Could you check a few things on this model? Use its own coordinates, in mm. A direction names the side the tool comes from. Give positions to 0.01 mm unless a question says otherwise; leave off trailing zeros. Write each loop counter-clockwise with the first axis right and the second up, starting at its lowest first coordinate (ties: lowest second). Pieces come first, ordered by that corner, then holes. Notation, with made-up numbers: (-38, 28) - (-17, 28) arc R36 cw to (-17, 62) - close; hole circle Ø2 at (89, 89). An arc over 180 degrees is marked (long way). Write item = value, one per line.
from build123d import *

# Parameters (mm, degrees)
F0_R            = 2.15265
F1_DEPTH        = 12.7
F2_R            = 2.15265
F3_REACH        = 42.6021136501
F6_R            = 3.96875
F7_DEPTH        = 9.525
F9_DEPTH        = 12.7
F9_COPIES_COUNT = 3
F9_COPIES_ANGLE = 180
F10_R           = 3.96875
F11_DEPTH       = 9.525


# Not quite as in the source:
# - a pattern or mirror of a feature is missing from the dataset's text; its kind, count and spacing are read off the source's solid


with BuildPart() as f1:
    # F0 (on Top) → F1 (new body)
    with BuildSketch(Plane.XY):
        with BuildLine():
            Line((3.96875, 14.2875), (0, 14.2875))
            Line((0, 14.2875), (-3.96875, 14.2875))
            Line((-3.96875, 14.2875), (-3.96875, 21.8677764859))
            ThreePointArc((-3.96875, 21.8677764859), (0, -22.225), (3.96875, 21.8677764859))
            Line((3.96875, 21.8677764859), (3.96875, 14.2875))
        make_face()
        with Locations((-11.7865861589, -11.7865861589)):
            Circle(F0_R, mode=Mode.SUBTRACT)
        with Locations((11.7865861589, -11.7865861589)):
            Circle(F0_R, mode=Mode.SUBTRACT)
        with Locations((-11.7865861589, 11.7865861589)):
            Circle(F0_R, mode=Mode.SUBTRACT)
        with BuildLine():
            ThreePointArc((0, 11.1125), (7.8577241059, 7.8577241059), (11.1125, 0))
            ThreePointArc((11.1125, 0), (-7.8577241059, -7.8577241059), (0, 11.1125))
        make_face(mode=Mode.SUBTRACT)
        with Locations((11.7865861589, 11.7865861589)):
            Circle(F0_R, mode=Mode.SUBTRACT)
    extrude(amount=F1_DEPTH)

    f3_end = f1.faces().sort_by_distance((0, -11.1125, 6.35))[0]
    # F2 (on face) → F3 (cut, up to a face of the model that its end follows)
    with BuildSketch(Plane(origin=(0, 14.2875, 0), x_dir=(-1, 0, 0), z_dir=(0, 1, 0))):
        with Locations((0, 6.35)):
            Circle(F2_R)
    f3_long = extrude(amount=-F3_REACH, mode=Mode.PRIVATE)
    add(split(f3_long, bisect_by=f3_end, keep=Keep.ALL, mode=Mode.PRIVATE).solids().sort_by_distance((0, 14.2875, 6.35))[0], mode=Mode.SUBTRACT)

    # F6 (on face) → F7 (cut, through all)
    with BuildSketch(Plane(origin=(0, 0, 0), x_dir=(1, 0, 0), z_dir=(0, 0, -1))):
        with Locations((11.7865861589, -11.7865861589)):
            Circle(F6_R)
        with Locations((-11.7865861589, 11.7865861589)):
            Circle(F6_R)
    extrude(amount=-F7_DEPTH, mode=Mode.SUBTRACT)

    # F8 (on face) → F9 (cut, through all)
    with BuildSketch(Plane(origin=(0, 0, 0), x_dir=(1, 0, 0), z_dir=(0, 0, -1))):
        with BuildLine():
            ThreePointArc((-17.3148424047, -11.229543123), (-15.8788163052, -8.0281867), (-12.8109235396, -6.3255746232))
            ThreePointArc((-12.8109235396, -6.3255746232), (-14.2875, 0), (-12.8109235396, 6.3255746232))
            ThreePointArc((-12.8109235396, 6.3255746232), (-15.8788163052, 8.0281867), (-17.3148424047, 11.229543123))
            ThreePointArc((-17.3148424047, 11.229543123), (-20.6375, 0), (-17.3148424047, -11.229543123))
        make_face()
    f9 = extrude(amount=-F9_DEPTH, mode=Mode.SUBTRACT)

    # F9_copies: F9 ×3 about axis
    f9_copies_axis = Axis((0, 0, 0), (0, 0, 1))
    for i in range(1, F9_COPIES_COUNT):
        add(f9.rotate(f9_copies_axis, i * F9_COPIES_ANGLE / (F9_COPIES_COUNT - 1)), mode=Mode.SUBTRACT)

    # F10 (on face) → F11 (cut, through all)
    with BuildSketch(Plane.XY.offset(12.7)):
        with Locations((11.7865861589, -11.7865861589)):
            Circle(F10_R)
        with Locations((-11.7865861589, 11.7865861589)):
            Circle(F10_R)
    extrude(amount=-F11_DEPTH, mode=Mode.SUBTRACT)


solid = f1.part
1. Thinking about a two-plate mould opening in X: for faces 1 (the face through (-0.921, -22.206, 6.261)), 2 (the face through (15.45, 13.31, 4.7)), 3 (the face through (-7, 10, 12.7)), which applies, pulls with the +X half, pulls with the -X half, needs draft (parallel to the pull), parting line crosses it, or undercut?
Filled sheet:
face_1 = parting line crosses it
face_2 = undercut
face_3 = needs draft
2. For pin 1 (6.5 mm diameter, centred on x = 11.79, y = 11.79, fed in from -Z) (3 decimals); pin 2 (4 mm diameter, centred on y = 19.5, z = 9, fed in from +X); pin 3 (6 mm diameter, centred on y = -15.5, z = 5, fed in from -X); pin 4 (3.5 mm diameter, centred on x = -11.79, y = -11.79, fed in from +Z), each with a flat end and sliding along its axis, tell me the tip position at first contact or that it passes through.
Filled sheet:
pin_1 = 9.525
pin_2 = 13.7
pin_3 = -18.38
pin_4 = through
3. I need wall thicknesses on line 1 (X direction, y = 2, z = 10); line 2 (X direction, y = -12, z = 10.75); line 3 (X direction, y = 7, z = 10.5). Which ranges of each line are inside material? Lowest first, please.
Filled sheet:
line_1 = -22.13 to -20.54, -14.15 to -10.93, 10.93 to 14.15, 20.54 to 22.13
line_2 = -18.71 to -13.93, -9.64 to 7.82, 15.75 to 18.71
line_3 = -21.09 to -19.41, -14.61 to -8.63, 8.63 to 14.61, 19.41 to 21.09
4. If we section it at A-A, the plane x = 16.5: Please give me the cut outline in (y, z), and give its area (3 significant figures).
Filled sheet:
outline = (-14.89, 0) - (-8.84, 0) - (-8.84, 12.7) - (-14.89, 12.7) - close; (8.84, 0) - (14.89, 0) - (14.89, 12.7) - (8.84, 12.7) - close
area = 154 mm2
5. Which directions (+Z, -Z, +X, -X, +Y, -Y) give clear straight access to the entire face, cutting with the end or side of a thin tool? Please do faces 4 (the face through (3.969, 18, 6)), 5 (the face through (13.5, 13.5, 9.525)), 6 (the face through (-10.63, -9.97, 11.09)).
Filled sheet:
face_4 = +Z, -Z, +Y
face_5 = -Z
face_6 = +Z, -Z
6. If we section it at C-C, the plane x = -7: Please give me the cut outline in (y, z), and give its area (3 significant figures).
Filled sheet:
outline = (-21.09, 0) - (-19.41, 0) - (-19.41, 12.7) - (-21.09, 12.7) - close; (-14.61, 0) - (-8.63, 0) - (-8.63, 12.7) - (-14.61, 12.7) - close; (8.63, 0) - (21.09, 0) - (21.09, 12.7) - (8.63, 12.7) - close
area = 256 mm2
7. If we section it at B-B, the plane z = 6.35: Count the separate pieces of the cut face and the enclosed holes in it, and give its area (3 significant figures).
Filled sheet:
separate_pieces = 1
enclosed_holes = 7
area = 569 mm2
